```python
from build123d import *

# Parameters (mm, degrees)
BOSS_EXTRUDE1_DEPTH = 1.6
SKETCH2_R           = 1.35
CUT_EXTRUDE1_DEPTH  = 87.467103571
SKETCH3_W           = 5
SKETCH3_H           = 51.3
BOSS_EXTRUDE2_DEPTH = 5.7


with BuildPart() as part:
    # Sketch1 → Boss-Extrude1 (new body)
    with BuildSketch(Plane(origin=(0, 0, 0), x_dir=(1, 0, 0), z_dir=(0, 1, 0))):
        with BuildLine():
            Line((3, 0), (54, 0))
            ThreePointArc((54, 0), (56.121320344, 0.878679656), (57, 3))
            Line((57, 3), (57, 62))
            ThreePointArc((57, 62), (56.121320344, 64.121320344), (54, 65))
            Line((54, 65), (3, 65))
            ThreePointArc((3, 65), (0.878679656, 64.121320344), (0, 62))
            Line((0, 62), (0, 3))
            ThreePointArc((0, 3), (0.878679656, 0.878679656), (3, 0))
        make_face()
    extrude(amount=BOSS_EXTRUDE1_DEPTH)

    # Sketch2 → Cut-Extrude1 (cut, through all)
    with BuildSketch(Plane(origin=(0, 1.6, 0), x_dir=(1, 0, 0), z_dir=(0, 1, 0))):
        with Locations(Location((4, 61.5, 0), (0, 0, 270))):
            Circle(SKETCH2_R)
        with Locations(Location((53, 61.5, 0), (0, 0, 270))):
            Circle(SKETCH2_R)
        with Locations(Location((53, 3.5, 0), (0, 0, 270))):
            Circle(SKETCH2_R)
        with Locations(Location((4, 3.5, 0), (0, 0, 270))):
            Circle(SKETCH2_R)
    extrude(amount=-CUT_EXTRUDE1_DEPTH, mode=Mode.SUBTRACT)

    # Sketch3 → Boss-Extrude2 (add)
    with BuildSketch(Plane.XZ):
        with Locations((53, -32.5)):
            Rectangle(SKETCH3_W, SKETCH3_H)
    extrude(amount=BOSS_EXTRUDE2_DEPTH)


solid = part.part
```
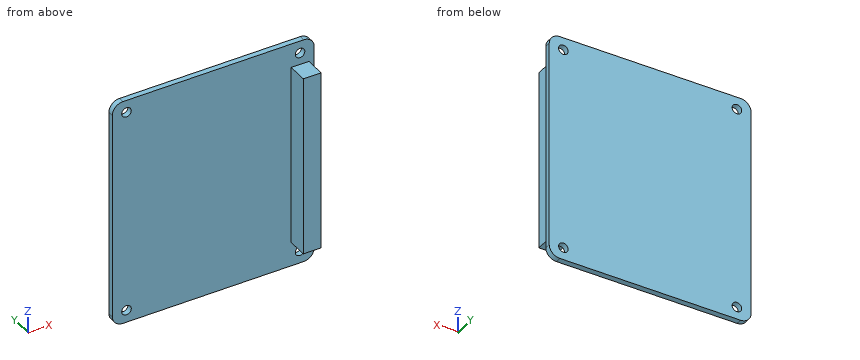
Geometry check sheet. Reference: the model listing, model coordinates, mm. Coordinates: 2 decimals unless noted, no trailing zeros. Write each loop counter-clockwise with the first axis right and the second up, starting at its lowest first coordinate (ties: lowest second). Pieces come first, ordered by that corner, then holes. Notation, with made-up numbers: M 71.5,56.25 L 119.5,56.25 A11 ccw 119.5,62.25 Z; hole C 74,84.25 d1. An arc over 180 degrees is marked long. Use one line per item in the form item = value. Start each with the question number.
1) Section check B-B on z = -22. Enter the section's corners in (x, y), and give its area (3 significant figures).
2) Section check D-D on y = -4.5. Enter the section's corners in (x, z).
3) Section check C-C on x = 28. Enter the section's corners in (y, z), and give its area (3 significant figures).
4) Thickness scan on probe 1 along X at (y, z) = (0.95, -3.5); probe 2 along Z at (x, y) = (5, 1); probe 3 along Y at (x, z) = (40.5, -50.5). Record the ranges inside material, lowest first. Write a range as from..to.
5) Go/stop test with flat-tipped pins: pin 1 Ø4 at (y, z) = (-2.5, -30) entering from +X; pin 2 Ø4 at (x, y) = (53.5, -2.5) entering from +Z; pin 3 Ø4 at (x, y) = (53, -4) entering from -Z; pin 4 Ø2 at (x, z) = (4, -61.5) entering from +Y. Record where each tip stops, or that it passes through.
6) Section check A-A on x = 4. Enter the section's corners in (y, z).
Responses:
q1.outline = M 0,0 L 50.5,0 L 50.5,-5.7 L 55.5,-5.7 L 55.5,0 L 57,0 L 57,1.6 L 0,1.6 Z
q1.area = 120 mm2
q2.outline = M 50.5,-58.15 L 55.5,-58.15 L 55.5,-6.85 L 50.5,-6.85 Z
q3.outline = M 0,-65 L 1.6,-65 L 1.6,0 L 0,0 Z
q3.area = 104 mm2
q4.probe_1 = 0..2.65, 5.35..51.65, 54.35..57
q4.probe_2 = -65..-62.41, -60.59..-4.41, -2.59..0
q4.probe_3 = 0..1.6
q5.pin_1 = 55.5
q5.pin_2 = -6.85
q5.pin_3 = -58.15
q5.pin_4 = through
q6.outline = M 0,-65 L 1.6,-65 L 1.6,-62.85 L 0,-62.85 Z; M 0,-60.15 L 1.6,-60.15 L 1.6,-4.85 L 0,-4.85 Z; M 0,-2.15 L 1.6,-2.15 L 1.6,0 L 0,0 Z
